CAD build for the part. Positions are in the model's coordinates, mm. Face numbers are marked on the shaded views. A direction names the side the tool comes from. Round coordinates to 2 decimals unless told otherwise and drop trailing zeros. Write each loop counter-clockwise with the first axis right and the second up, starting at its lowest first coordinate (ties: lowest second). Pieces come first, ordered by that corner, then holes. Notation, with made-up numbers: (29.25, -8) - (35.25, -8) arc R12 cw to (35.25, 0) - close; hole circle Ø11 at (86, 8.5). An arc over 180 degrees is marked (long way). Use one line per item in the form item = value. Start each with the question number.
Item 1: Band-saw the part on A-A, the plane x = 15.7. Give the number of separate pieces and of enclosed holes in the cut face, and give its area (3 significant figures).
Item 2: Band-saw the part on D-D, the plane y = -39. List the corners of the cut face in (x, z).
Item 3: Tool access for the marked faces 1, 2, 3 and 4: list every direction of +Z, -Z, +X, -X, +Y, -Y with a clear straight run to the whole face (end or side of a thin tool).
Item 4: Pull direction Z, two halves, no side cores. Call the marked faces 5, 6 and 7: +Z half, -Z half, draft (parallel to the pull), parting line (faces both ways), or undercut.
Item 5: Drill centre lines: L1, parallel to Y at x = 5.7, z = 1.25; L2, parallel to X at y = -49, z = 0.8; L3, parallel to X at y = -49, z = 16.3. Where is each one in solid material? Low to high.
Item 6: Pin check, flat tips, straight feed: pin 1 (10 mm diameter, centred on y = -19.5, z = 12.5, fed in from +X); pin 2 (1.5 mm diameter, centred on x = -5.5, y = -28.5, fed in from +Z); pin 3 (6 mm diameter, centred on y = -28, z = 6.5, fed in from -X). Stop position of each tip, or through.
Item 7: Band-saw the part on C-C, the plane x = 29. List the corners of the cut face in (y, z), and give its area (3 significant figures).
Item 8: Band-saw the part on B-B, the plane z = 11.5. List the corners of the cut face in (x, y).
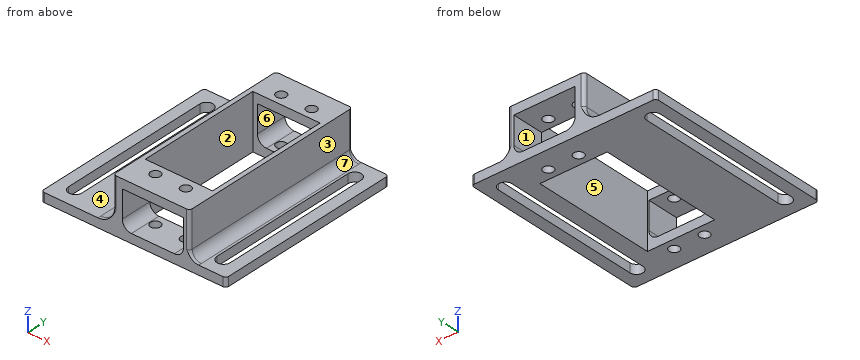
from build123d import *

# Parameters (mm, degrees)
SKETCH_1_W          = 60.8
SKETCH_1_H          = 62
EXTRUDE_1_DEPTH     = 3
SKETCH_2_W          = 25.15
SKETCH_2_H          = 62
SKETCH_2_R          = 1.65
EXTRUDE_2_DEPTH     = 15
CUT_EXTRUDE_START   = -45
SKETCH_4_R          = 1.65
SKETCH_4_W          = 22.15
SKETCH_4_H          = 41
CUT_EXTRUDE_4_DEPTH = 45
FILLET_1_R          = 1
FILLET_2_R          = 5
SKETCH_5_W          = 20.15
SKETCH_5_H          = 12
CUT_EXTRUDE_5_DEPTH = 70
FILLET_3_R          = 3
FILLET_4_R          = 3


with BuildPart() as part:
    # 草图1 → 凸台-拉伸1 (new body)
    with BuildSketch(Plane.XY):
        with Locations((4.6, -25)):
            Rectangle(SKETCH_1_W, SKETCH_1_H)
        with BuildLine():
            Line((26.8, 0), (26.8, -50))
            ThreePointArc((26.8, -50), (29, -52.2), (31.2, -50))
            Line((31.2, -50), (31.2, 0))
            ThreePointArc((31.2, 0), (29, 2.2), (26.8, 0))
        make_face(mode=Mode.SUBTRACT)
        with BuildLine():
            Line((-22, 0), (-22, -50))
            ThreePointArc((-22, -50), (-19.8, -52.2), (-17.6, -50))
            Line((-17.6, -50), (-17.6, 0))
            ThreePointArc((-17.6, 0), (-19.8, 2.2), (-22, 0))
        make_face(mode=Mode.SUBTRACT)
    extrude(amount=EXTRUDE_1_DEPTH)

    # 草图2 → 凸台-拉伸2 (add)
    with BuildSketch(Plane.XY.offset(3)):
        with Locations((10.425, -25)):
            Rectangle(SKETCH_2_W, SKETCH_2_H)
        with Locations((5.7, -1)):
            Circle(SKETCH_2_R, mode=Mode.SUBTRACT)
        with Locations((15.7, -1)):
            Circle(SKETCH_2_R, mode=Mode.SUBTRACT)
        with Locations((15.7, -49)):
            Circle(SKETCH_2_R, mode=Mode.SUBTRACT)
        with Locations((5.7, -49)):
            Circle(SKETCH_2_R, mode=Mode.SUBTRACT)
    extrude(amount=EXTRUDE_2_DEPTH)

    # 草图4 → 切除-拉伸4 (cut)
    with BuildSketch(Plane.XY.offset(18).offset(CUT_EXTRUDE_START)):
        with Locations((5.7, -1)):
            Circle(SKETCH_4_R)
        with Locations((5.7, -49)):
            Circle(SKETCH_4_R)
        with Locations((15.7, -49)):
            Circle(SKETCH_4_R)
        with Locations((15.7, -1)):
            Circle(SKETCH_4_R)
        with Locations((10.425, -25)):
            Rectangle(SKETCH_4_W, SKETCH_4_H)
    extrude(amount=CUT_EXTRUDE_4_DEPTH, mode=Mode.SUBTRACT)

    # 圆角1
    fillet_1_edges = [part.edges().sort_by_distance(p)[0] for p in [
        (-2.15, 6, 10.5),
        (-2.15, -56, 10.5),
        (23, -56, 10.5),
        (23, 6, 10.5),
        (-25.8, 6, 1.5),
        (35, 6, 1.5),
        (35, -56, 1.5),
        (-25.8, -56, 1.5),
    ]]
    fillet(fillet_1_edges, radius=FILLET_1_R)

    # 圆角2
    # the kernel refuses this fillet: 5 mm, written as the material it adds along each edge
    with BuildSketch(Plane(origin=(-2.15, -55, 3), x_dir=(0, 0, 1), z_dir=(0, 1, 0))) as fillet_2_piece_1:
        with BuildLine():
            CenterArc((FILLET_2_R, -FILLET_2_R), FILLET_2_R, 90, 90)
            Line((0, -FILLET_2_R), (0, 0))
            Line((0, 0), (FILLET_2_R, 0))
        make_face()
    extrude(amount=60)
    with BuildSketch(Plane(origin=(-1.15, 5, 3), x_dir=(-0.9999802608561372, -0.00628314396555929, 0), z_dir=(-0.00628314396555929, 0.9999802608561372, 0))) as fillet_2_piece_2_section:
        with BuildLine():
            CenterArc((-1 - FILLET_2_R, FILLET_2_R), FILLET_2_R, 270, 90)
            Line((-1 - FILLET_2_R, 0), (-1, 0))
            Line((-1, 0), (-1, FILLET_2_R))
        make_face()
    fillet_2_piece_2 = revolve(axis=Axis((-1.15, 5, 3), (0, 0, 1)), revolution_arc=359.64, mode=Mode.PRIVATE)
    fillet_2_piece_2 = split(fillet_2_piece_2, bisect_by=Plane(origin=(-1.917475006, 6, 5.017645517), z_dir=(0, -1, 0)), keep=Keep.TOP, mode=Mode.PRIVATE)
    add(fillet_2_piece_2)
    with BuildSketch(Plane(origin=(-1.15, -55, 3), x_dir=(-0.9999802608561372, 0.006283143965561067, 0), z_dir=(-0.006283143965561067, -0.9999802608561372, 0))) as fillet_2_piece_3_section:
        with BuildLine():
            CenterArc((-1 - FILLET_2_R, -FILLET_2_R), FILLET_2_R, 0, 90)
            Line((-1 - FILLET_2_R, 0), (-1, 0))
            Line((-1, 0), (-1, -FILLET_2_R))
        make_face()
    fillet_2_piece_3 = revolve(axis=Axis((-1.15, -55, 3), (0, 0, -1)), revolution_arc=359.64, mode=Mode.PRIVATE)
    fillet_2_piece_3 = split(fillet_2_piece_3, bisect_by=Plane(origin=(-1.917475041, -56, 5.017645533), z_dir=(0, 1, 0)), keep=Keep.TOP, mode=Mode.PRIVATE)
    add(fillet_2_piece_3)

    # 草图5 → 切除-拉伸5 (cut)
    with BuildSketch(Plane(origin=(0, -56, 0), x_dir=(-1, 0, 0), z_dir=(0, -1, 0))):
        with Locations((-10.925, -9)):
            Rectangle(SKETCH_5_W, SKETCH_5_H)
    extrude(amount=-CUT_EXTRUDE_5_DEPTH, mode=Mode.SUBTRACT)

    # 圆角3
    fillet_3_edges = [part.edges().sort_by_distance(p)[0] for p in [
        (0.85, 0.75, 3),
        (0.85, -50.75, 3),
        (21, 0.75, 3),
        (21, -50.75, 3),
    ]]
    fillet(fillet_3_edges, radius=FILLET_3_R)

    # 圆角4
    # the kernel refuses this fillet: 3 mm, written as the material it adds along each edge
    with BuildSketch(Plane(origin=(23, 5, 3), x_dir=(1, 0, 0), z_dir=(0, -1, 0))) as fillet_4_piece_1:
        with BuildLine():
            CenterArc((FILLET_4_R, FILLET_4_R), FILLET_4_R, 180, 90)
            Line((0, FILLET_4_R), (0, 0))
            Line((0, 0), (FILLET_4_R, 0))
        make_face()
    extrude(amount=60)
    with BuildSketch(Plane(origin=(22, 5, 3), x_dir=(0.9999802608561372, -0.0062831439655584, 0), z_dir=(0.0062831439655584, 0.9999802608561372, 0))) as fillet_4_piece_2_section:
        with BuildLine():
            CenterArc((-1 - FILLET_4_R, -FILLET_4_R), FILLET_4_R, 0, 90)
            Line((-1, -FILLET_4_R), (-1, 0))
            Line((-1, 0), (-1 - FILLET_4_R, 0))
        make_face()
    fillet_4_piece_2 = revolve(axis=Axis((22, 5, 3), (0, 0, -1)), revolution_arc=359.64, mode=Mode.PRIVATE)
    fillet_4_piece_2 = split(fillet_4_piece_2, bisect_by=Plane(origin=(22.764056833, 6, 4.135633633), z_dir=(0, -1, 0)), keep=Keep.TOP, mode=Mode.PRIVATE)
    add(fillet_4_piece_2)
    with BuildSketch(Plane(origin=(22, -55, 3), x_dir=(0.9999802608561372, 0.006283143965561065, 0), z_dir=(0.006283143965561065, -0.9999802608561372, 0))) as fillet_4_piece_3_section:
        with BuildLine():
            CenterArc((-1 - FILLET_4_R, FILLET_4_R), FILLET_4_R, 270, 90)
            Line((-1 - FILLET_4_R, 0), (-1, 0))
            Line((-1, 0), (-1, FILLET_4_R))
        make_face()
    fillet_4_piece_3 = revolve(axis=Axis((22, -55, 3), (0, 0, 1)), revolution_arc=359.64, mode=Mode.PRIVATE)
    fillet_4_piece_3 = split(fillet_4_piece_3, bisect_by=Plane(origin=(22.76405677, -56, 4.135633616), z_dir=(0, 1, 0)), keep=Keep.TOP, mode=Mode.PRIVATE)
    add(fillet_4_piece_3)


solid = part.part
Determined:
q1.separate_pieces = 8
q1.enclosed_holes = 0
q1.area = 86.4 mm²
q2.outline = (-25.8, 0) - (-22, 0) - (-22, 3) - (-25.8, 3) - close; (-17.6, 0) - (-0.65, 0) - (-0.65, 18) - (-2.15, 18) - (-2.15, 8) arc R5 cw to (-7.15, 3) - (-17.6, 3) - close; (21.5, 0) - (26.8, 0) - (26.8, 3) - (26, 3) arc R3 cw to (23, 6) - (23, 18) - (21.5, 18) - close; (31.2, 0) - (35, 0) - (35, 3) - (31.2, 3) - close
q3.face_1 = +Y, -Y
q3.face_2 = +Z, -Z
q3.face_3 = +Z, +X, +Y, -Y
q3.face_4 = +Z, -X, +Y, -Y
q4.face_5 = draft
q4.face_6 = undercut
q4.face_7 = +Z half
q5.L1 = -56 to -50.65, -47.35 to -45.5, -4.5 to -2.65, 0.65 to 6
q5.L2 = -25.8 to -22, -17.6 to 4.05, 7.35 to 14.05, 17.35 to 26.8, 31.2 to 35
q5.L3 = -2.15 to 4.05, 7.35 to 14.05, 17.35 to 23
q6.pin_1 = 23
q6.pin_2 = 3.61
q6.pin_3 = -4.97
q7.outline = (-56, 0) - (-52.2, 0) - (-52.2, 3) - (-56, 3) - close; (2.2, 0) - (6, 0) - (6, 3) - (2.2, 3) - close
q7.area = 22.8 mm²
q8.outline = (-2.15, -55) arc R1 ccw to (-1.15, -56) - (0.85, -56) - (0.85, -45.5) - (-0.65, -45.5) - (-0.65, -4.5) - (0.85, -4.5) - (0.85, 6) - (-1.15, 6) arc R1 ccw to (-2.15, 5) - close; (21, -56) - (22, -56) arc R1 ccw to (23, -55) - (23, 5) arc R1 ccw to (22, 6) - (21, 6) - (21, -4.5) - (21.5, -4.5) - (21.5, -45.5) - (21, -45.5) - close
